Check sheet for the modelled part. Datum: model origin and axes. Units: mm. Face numbers are marked on the shaded views. A direction names the side the tool comes from. Give positions to 0.01 mm unless a question says otherwise; leave off trailing zeros. Loops run counter-clockwise (first coordinate to the right, second up) from the corner with the lowest first, then second, coordinate; pieces in that order, holes last. Notation, with made-up numbers: (-33, -31.75) - (25, -31.75) arc R17 cw to (25, -3.75) - close; hole circle Ø2 at (33.25, -24). An arc over 180 degrees is marked (long way). Use one line per item in the form item = value.
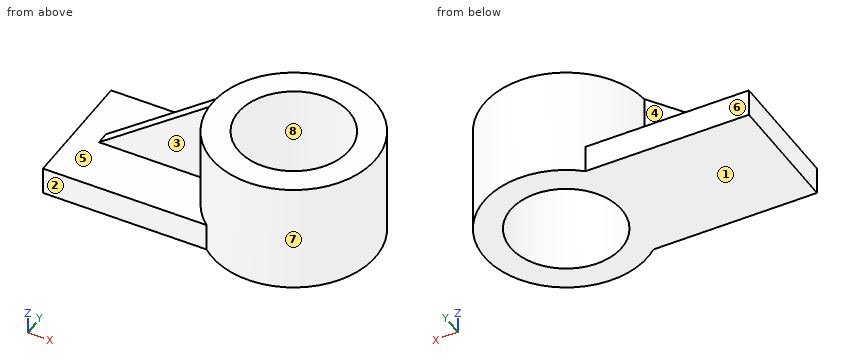
from build123d import *

# Parameters (mm, degrees)
F0_W      = 123.794436
F0_H      = 57.333368
F1_DEPTH  = 12.7
F2_R      = 37.794385
F3_DEPTH  = 50.8
F4_R      = 25.640341
F5_DEPTH  = 50.8
F6_W      = 100.285656
F6_H      = 5.836856
F7_DEPTH  = 38.1
F8_R      = 25.640341
F9_DEPTH  = 50.8
F11_DEPTH = 25.4


with BuildPart() as f1:
    # F0 (on Top) → F1 (new body)
    with BuildSketch(Plane.XY):
        Rectangle(F0_W, F0_H)
    extrude(amount=F1_DEPTH)

    # F2 (on Top) → F3 (join)
    with BuildSketch(Plane.XY):
        with Locations((38.222246, 0)):
            Circle(F2_R)
    extrude(amount=F3_DEPTH)

    # F4 (on face) → F5 (cut)
    with BuildSketch(Plane.XY.offset(50.8)):
        with Locations((38.222246, 0)):
            Circle(F4_R)
    extrude(amount=-F5_DEPTH, mode=Mode.SUBTRACT)

    # F6 (on face) → F7 (join)
    with BuildSketch(Plane.XY.offset(12.7)):
        Rectangle(F6_W, F6_H)
    extrude(amount=F7_DEPTH)

    # F8 (on face) → F9 (cut)
    with BuildSketch(Plane.XY.offset(50.8)):
        with Locations((38.222246, 0)):
            Circle(F8_R)
    extrude(amount=-F9_DEPTH, mode=Mode.SUBTRACT)

    # F10 (on face) → F11 (cut)
    with BuildSketch(Plane.XZ.offset(2.918428)):
        Polygon((-50.142828, 12.7), (0.540708, 50.8), (-50.142828, 50.8), align=None)
    extrude(amount=-F11_DEPTH, mode=Mode.SUBTRACT)


solid = f1.part
Item 1: Gauge pin test, flat ends, axial feed: P1, Ø5, axis at y = -1.5, z = 20, coming from the -X side; P2, Ø8, axis at x = -32, y = 21, coming from the -Z side; P3, Ø11.5, axis at x = -33, z = 28.5, coming from the -Y side; P4, Ø14, axis at x = -43, z = 8.5, coming from the -Y side. Record the tip position at first contact, or that the pin passes through.
Answer block:
P1 = -43.76
P2 = 0
P3 = -2.92
P4 = -28.67
Item 2: Section check C-C on z = 29. Record the boundary of the cut face in (x, y).
Answer block:
outline = (-28.46, -2.92) - (0.54, -2.92) arc R37.79 ccw (long way) to (0.54, 2.92) - (-28.46, 2.92) - close; hole circle Ø51.28 at (38.22, 0)
Item 3: Section check A-A on y = 0. Record the boundary of the cut face in (x, z), then the cut area to 3 significant figures.
Answer block:
outline = (-61.9, 0) - (12.58, 0) - (12.58, 50.8) - (0.54, 50.8) - (-50.14, 12.7) - (-61.9, 12.7) - close; (63.86, 0) - (76.02, 0) - (76.02, 50.8) - (63.86, 50.8) - close
area = 2,990 mm2
Item 4: Access from +Z, -Z, +X, -X, +Y, -Y to the whole of each face (thin tool, end or side, straight path). Record for the marked faces 1, 2, 3, 4 and 5.
Answer block:
face_1 = -Z, +X, -X, +Y, -Y
face_2 = +Z, -Z, -X, -Y
face_3 = +Z, -X, -Y
face_4 = +Z, -X, +Y
face_5 = +Z, -X
Item 5: Mould release check, pull along X, two halves, no side actions. Record for the marked faces 6, 7 and 8: released by +X, released by -X, zero draft, split by the parting line, or undercut.
Answer block:
face_6 = zero draft
face_7 = split by the parting line
face_8 = undercut
Item 6: Section check B-B on x = 48. Record the boundary of the cut face in (y, z).
Answer block:
outline = (-36.51, 0) - (-23.7, 0) - (-23.7, 50.8) - (-36.51, 50.8) - close; (23.7, 0) - (36.51, 0) - (36.51, 50.8) - (23.7, 50.8) - close
Item 7: Thickness scan on L1, parallel to Z at x = -9.5, y = -14; L2, parallel to Y at x = 59, z = 6; L3, parallel to X at y = 0.5, z = 32. Record the ranges inside material, lowest first.
Answer block:
L1 = 0 to 12.7
L2 = -31.57 to -15.02, 15.02 to 31.57
L3 = -24.47 to 12.59, 63.86 to 76.01
Item 8: Section check D-D on x = -31. Record the boundary of the cut face in (y, z).
Answer block:
outline = (-28.67, 0) - (28.67, 0) - (28.67, 12.7) - (2.92, 12.7) - (2.92, 27.09) - (-2.92, 27.09) - (-2.92, 12.7) - (-28.67, 12.7) - close
